from build123d import *

# Parameters (mm, degrees)
FONDO_START                   = -54
SK_FONDO_W                    = 220
SK_FONDO_H                    = 220
FONDO_DEPTH                   = 4
PASANTES_M4_SEPARADORES_START = -54
SK_PASANTES_M4_SEPARADORES_R  = 2.25
PASANTES_M4_SEPARADORES_DEPTH = 4
AVELLANADO_M4_START           = -54
SK_AVELLANADO_M4_R            = 4.2
AVELLANADO_M4_DEPTH           = 2.5
PASANTES_M2_5_RPI_START       = -54
SK_PASANTES_M2_5_RPI_R        = 1.45
PASANTES_M2_5_RPI_DEPTH       = 4
AVELLANADO_M2_5_START         = -54
SK_AVELLANADO_M2_5_R          = 2.5
AVELLANADO_M2_5_DEPTH         = 1.5
AGUJEROS_ANCLAJE_START        = -54
SK_AGUJEROS_ANCLAJE_R         = 3.3
AGUJEROS_ANCLAJE_DEPTH        = 4


with BuildPart() as part:
    # Sk_Fondo → Fondo (new body)
    with BuildSketch(Plane.XY.offset(FONDO_START)):
        Rectangle(SK_FONDO_W, SK_FONDO_H)
    extrude(amount=FONDO_DEPTH)

    # Sk_Pasantes_M4_separadores → Pasantes_M4_separadores (cut)
    with BuildSketch(Plane.XY.offset(PASANTES_M4_SEPARADORES_START)):
        with Locations((-95, -95)):
            Circle(SK_PASANTES_M4_SEPARADORES_R)
        with Locations((-95, 95)):
            Circle(SK_PASANTES_M4_SEPARADORES_R)
        with Locations((95, -95)):
            Circle(SK_PASANTES_M4_SEPARADORES_R)
        with Locations((95, 95)):
            Circle(SK_PASANTES_M4_SEPARADORES_R)
    extrude(amount=PASANTES_M4_SEPARADORES_DEPTH, mode=Mode.SUBTRACT)

    # Sk_Avellanado_M4 → Avellanado_M4 (cut)
    with BuildSketch(Plane.XY.offset(AVELLANADO_M4_START)):
        with Locations((-95, -95)):
            Circle(SK_AVELLANADO_M4_R)
        with Locations((-95, 95)):
            Circle(SK_AVELLANADO_M4_R)
        with Locations((95, -95)):
            Circle(SK_AVELLANADO_M4_R)
        with Locations((95, 95)):
            Circle(SK_AVELLANADO_M4_R)
    extrude(amount=AVELLANADO_M4_DEPTH, mode=Mode.SUBTRACT)

    # Sk_Pasantes_M2-5_RPi → Pasantes_M2-5_RPi (cut)
    with BuildSketch(Plane.XY.offset(PASANTES_M2_5_RPI_START)):
        with Locations((-13.5, -24.5)):
            Circle(SK_PASANTES_M2_5_RPI_R)
        with Locations((-13.5, 24.5)):
            Circle(SK_PASANTES_M2_5_RPI_R)
        with Locations((-71.5, -24.5)):
            Circle(SK_PASANTES_M2_5_RPI_R)
        with Locations((-71.5, 24.5)):
            Circle(SK_PASANTES_M2_5_RPI_R)
    extrude(amount=PASANTES_M2_5_RPI_DEPTH, mode=Mode.SUBTRACT)

    # Sk_Avellanado_M2-5 → Avellanado_M2-5 (cut)
    with BuildSketch(Plane.XY.offset(AVELLANADO_M2_5_START)):
        with Locations((-13.5, -24.5)):
            Circle(SK_AVELLANADO_M2_5_R)
        with Locations((-13.5, 24.5)):
            Circle(SK_AVELLANADO_M2_5_R)
        with Locations((-71.5, -24.5)):
            Circle(SK_AVELLANADO_M2_5_R)
        with Locations((-71.5, 24.5)):
            Circle(SK_AVELLANADO_M2_5_R)
    extrude(amount=AVELLANADO_M2_5_DEPTH, mode=Mode.SUBTRACT)

    # Sk_Agujeros_anclaje → Agujeros_anclaje (cut)
    with BuildSketch(Plane.XY.offset(AGUJEROS_ANCLAJE_START)):
        with Locations((-100, -40)):
            Circle(SK_AGUJEROS_ANCLAJE_R)
        with Locations((-100, 40)):
            Circle(SK_AGUJEROS_ANCLAJE_R)
        with Locations((100, -40)):
            Circle(SK_AGUJEROS_ANCLAJE_R)
        with Locations((100, 40)):
            Circle(SK_AGUJEROS_ANCLAJE_R)
    extrude(amount=AGUJEROS_ANCLAJE_DEPTH, mode=Mode.SUBTRACT)


solid = part.part
Could you check a few things on this model? Use its own coordinates, in mm. A direction names the side the tool comes from. Round coordinates to 2 decimals unless told otherwise and drop trailing zeros.
Q1. Thinking about a two-plate mould opening in X: for faces 3 (the face through (-98.226, -37.217, -52.028)), 4 (the face through (-2, 2, -50)), which applies, released by +X, released by -X, zero draft, split by the parting line, or undercut?
Geometry says:
face 3: undercut
face 4: zero draft
Q2. I'm going to push flat-ended pins straight in: P1, Ø7, axis at x = 95, y = -95, coming from the -Z side; P2, Ø5.5, axis at x = 100, y = -40, coming from the -Z side; P3, Ø4, axis at x = -13.5, y = 24.5, coming from the -Z side. Where does each tip first touch, or does it pass through?
Geometry says:
P1: stops at z = -51.5
P2: passes through
P3: stops at z = -52.5
Q3. Which directions (+Z, -Z, +X, -X, +Y, -Y) give clear straight access to the entire face, cutting with the end or side of a thin tool? Please do faces 1 (the face through (-98.226, 42.783, -52.028)), 2 (the face through (-13.83, 26.98, -53.26)).
Geometry says:
face 1: +Z, -Z
face 2: -Z
Q4. Please list where these lines run through material, in increasing order: probe 1 along Y at (x, z) = (-95, -50.5); probe 2 along Y at (x, z) = (-100, -50.8); probe 3 along X at (y, z) = (38, -52.3).
Geometry says:
probe 1: y = -110 to -97.25, -92.75 to 92.75, 97.25 to 110
probe 2: y = -110 to -43.3, -36.7 to 36.7, 43.3 to 110
probe 3: x = -110 to -102.62, -97.38 to 97.38, 102.62 to 110
